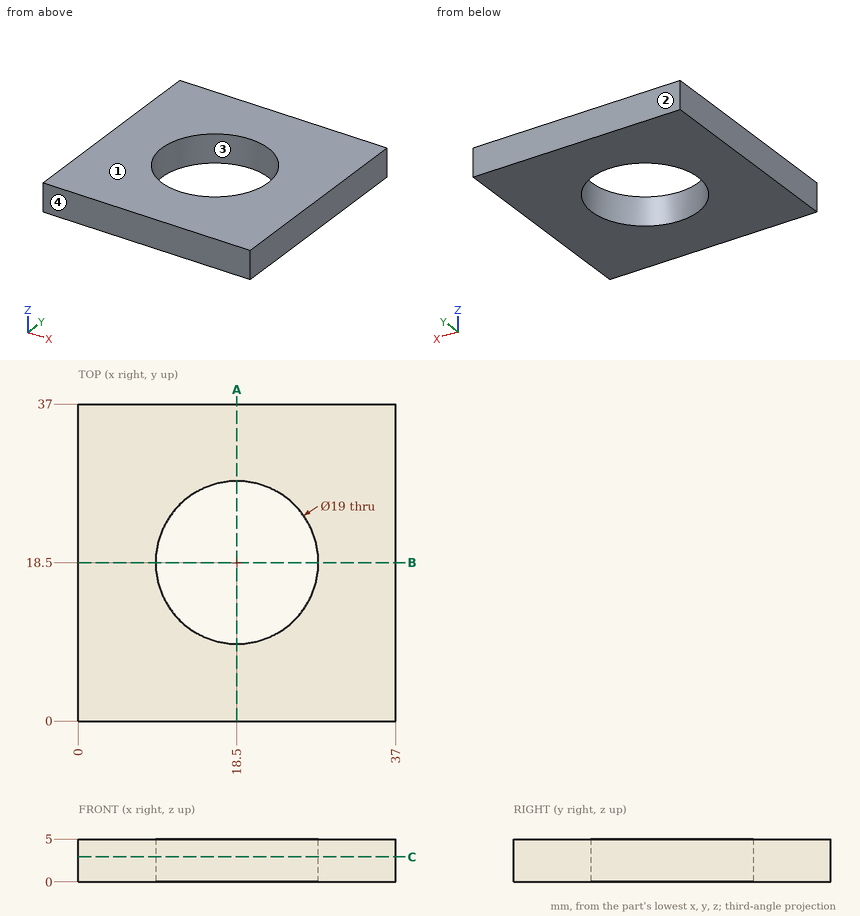
Print and shaded views of the part. All mm, measured from the part's lowest x, y and z. Coordinates: 2 decimals unless noted, no trailing zeros. Write each loop counter-clockwise with the first axis right and the second up, starting at its lowest first coordinate (ties: lowest second). Pieces come first, ordered by that corner, then holes. Notation, with made-up numbers: (84, 36.25) - (118, 36.25) arc R11 ccw to (118, 40.25) - close; hole circle Ø1 at (2.5, 85). An arc over 180 degrees is marked (long way). One line per question, with ' | ' between items. Start each with the question number.
Q1. Pull direction Y, two halves, no side cores. Call the marked faces 1, 2, 3 and 4: pulls with the +Y half, pulls with the -Y half, needs draft (parallel to the pull), parting line crosses it, or undercut.
Q2. Cut at A-A, the plane x = 18.5. List the corners of the cut face in (y, z), then the cut area to 3 significant figures.
Q3. Cut at C-C, the plane z = 2.9. List the corners of the cut face in (x, y), then the cut area to 3 significant figures.
Q4. Drill centre lines: line 1 (Y direction, x = 18.5, z = 3); line 2 (Y direction, x = 14, z = 4.1); line 3 (X direction, y = 16.5, z = 1.5). Where is each one in solid material? Low to high. Write a range as [from, to].
Answer below:
1) face 1: needs draft | face 2: pulls with the +Y half | face 3: undercut | face 4: pulls with the -Y half
2) outline: (0, 0) - (9, 0) - (9, 5) - (0, 5) - close; (28, 0) - (37, 0) - (37, 5) - (28, 5) - close | area: 90.0 mm^2
3) outline: (0, 0) - (37, 0) - (37, 37) - (0, 37) - close; hole circle Ø19 at (18.5, 18.5) | area: 1,090 mm^2
4) line 1: [0, 9], [28, 37] | line 2: [0, 10.13], [26.87, 37] | line 3: [0, 9.21], [27.79, 37]
